For this review, take the finished solid that the model builds, in its own axes (mm). Face numbers are marked on the shaded views. A direction names the side the tool comes from. Round coordinates to 2 decimals unless told otherwise and drop trailing zeros. Loops run counter-clockwise (first coordinate to the right, second up) from the corner with the lowest first, then second, coordinate; pieces in that order, holes last.
1. Tool access review of the marked faces 1, 2 and 3: name each direction out of +Z, -Z, +X, -X, +Y, -Y from which nothing blocks a thin tool from reaching the whole face with its end or side.
2. Clearance check with flat-ended pins moving along their axes: pin 1 Ø1 at (x, y) = (-14.5, 4.5) entering from +Z; pin 2 Ø0.6 at (x, z) = (8, -15.5) entering from +Y; pin 3 Ø12 at (x, z) = (2.5, 13) entering from +Y. State where each tip first meets the part, or that it passes through.
3. Consider section A-A on z = 17.5. State the section outline as (x, y) points, then the cut area to 3 significant figures.
4. To check wall thickness, follow line 1 along X through (y, z) = (18, -0.5); line 2 along Y through (x, z) = (9, 11); line 3 along X through (y, z) = (3.35, 17.5). State the ranges of each line that lie inside material, in increasing order.
5. Consider section D-D on z = -17.5. State how many separate pieces and enclosed holes the cut face has, then the cut area to 3 significant figures.
6. Consider section C-C on z = 5.5. State the section outline as (x, y) points.
7. Draft analysis for pull direction X (two halves, no side actions). For the marked faces 4, 5, 6 and 7, state which applies: released by +X, released by -X, zero draft, split by the parting line, or undercut.
8. Consider section B-B on y = 2.5. State the section outline as (x, z) points, then the cut area to 3 significant figures.
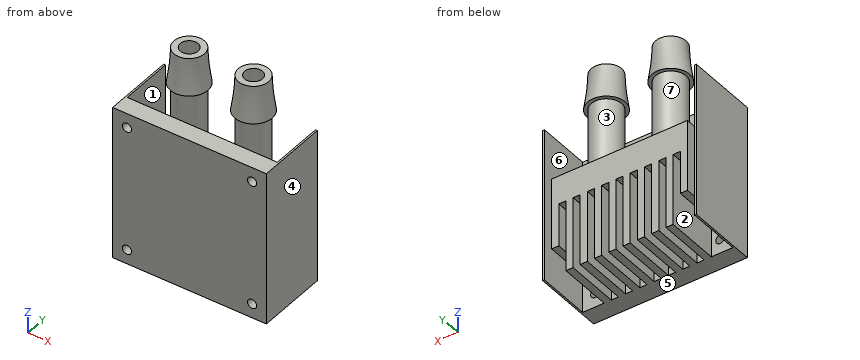
from build123d import *

# Parameters (mm, degrees)
SKETCH1_W               = 43
SKETCH1_H               = 43
BOSS_EXTRUDE1_DEPTH     = 20
SKETCH2_W               = 2
SKETCH2_H               = 15
CUT_EXTRUDE1_DEPTH      = 20
LPATTERN1_COUNT         = 6
LPATTERN1_PITCH         = 4
MIRROR1_COPY_1_SKETCH_W = 2
MIRROR1_COPY_1_SKETCH_H = 15
MIRROR1_COPY_1_DEPTH    = 20
MIRROR1_COPY_2_SKETCH_W = 2
MIRROR1_COPY_2_SKETCH_H = 15
MIRROR1_COPY_2_DEPTH    = 20
MIRROR1_COPY_3_SKETCH_W = 2
MIRROR1_COPY_3_SKETCH_H = 15
MIRROR1_COPY_3_DEPTH    = 20
MIRROR1_COPY_4_SKETCH_W = 2
MIRROR1_COPY_4_SKETCH_H = 15
MIRROR1_COPY_4_DEPTH    = 20
MIRROR1_COPY_5_SKETCH_W = 2
MIRROR1_COPY_5_SKETCH_H = 15
MIRROR1_COPY_5_DEPTH    = 20
MIRROR1_COPY_6_SKETCH_W = 2
MIRROR1_COPY_6_SKETCH_H = 15
MIRROR1_COPY_6_DEPTH    = 20
SKETCH7_W               = 2
SKETCH7_H               = 15
CUT_EXTRUDE6_DEPTH      = 38.299463803
SKETCH8_W               = 38
SKETCH8_H               = 15
CUT_EXTRUDE7_DEPTH      = 15
SKETCH9_R               = 4.25
BOSS_EXTRUDE2_DEPTH     = 20
SKETCH12_R              = 2.5
CUT_EXTRUDE8_DEPTH      = 35
SKETCH13_R              = 1.27
CUT_EXTRUDE9_DEPTH      = 47.845490789
SKETCH14_W              = 2
SKETCH14_H              = 8
CUT_EXTRUDE10_DEPTH     = 15


with BuildPart() as part:
    # Sketch1 → Boss-Extrude1 (new body)
    with BuildSketch(Plane(origin=(0, 0, 0), x_dir=(1, 0, 0), z_dir=(0, 1, 0))):
        Rectangle(SKETCH1_W, SKETCH1_H)
    extrude(amount=BOSS_EXTRUDE1_DEPTH)

    # Sketch2 → Cut-Extrude1 (cut)
    with BuildSketch(Plane(origin=(0, 0, -21.5), x_dir=(-1, 0, 0), z_dir=(0, 0, -1))):
        with Locations((0, 12.5)):
            Rectangle(SKETCH2_W, SKETCH2_H)
    cut_extrude1 = extrude(amount=-CUT_EXTRUDE1_DEPTH, mode=Mode.SUBTRACT)

    # LPattern1: Cut-Extrude1 ×6
    with Locations(*[(i * LPATTERN1_PITCH, 0, 0) for i in range(1, LPATTERN1_COUNT)]):
        add(cut_extrude1, mode=Mode.SUBTRACT)

    # Mirror1 copy 1 sketch → Mirror1 copy 1 (cut)
    with BuildSketch(Plane(origin=(-4, 0, -21.5), x_dir=(1, 0, 0), z_dir=(0, 0, -1))):
        with Locations((0, -12.5)):
            Rectangle(MIRROR1_COPY_1_SKETCH_W, MIRROR1_COPY_1_SKETCH_H)
    extrude(amount=-MIRROR1_COPY_1_DEPTH, mode=Mode.SUBTRACT)

    # Mirror1 copy 2 sketch → Mirror1 copy 2 (cut)
    with BuildSketch(Plane(origin=(-8, 0, -21.5), x_dir=(1, 0, 0), z_dir=(0, 0, -1))):
        with Locations((0, -12.5)):
            Rectangle(MIRROR1_COPY_2_SKETCH_W, MIRROR1_COPY_2_SKETCH_H)
    extrude(amount=-MIRROR1_COPY_2_DEPTH, mode=Mode.SUBTRACT)

    # Mirror1 copy 3 sketch → Mirror1 copy 3 (cut)
    with BuildSketch(Plane(origin=(-12, 0, -21.5), x_dir=(1, 0, 0), z_dir=(0, 0, -1))):
        with Locations((0, -12.5)):
            Rectangle(MIRROR1_COPY_3_SKETCH_W, MIRROR1_COPY_3_SKETCH_H)
    extrude(amount=-MIRROR1_COPY_3_DEPTH, mode=Mode.SUBTRACT)

    # Mirror1 copy 4 sketch → Mirror1 copy 4 (cut)
    with BuildSketch(Plane(origin=(-16, 0, -21.5), x_dir=(1, 0, 0), z_dir=(0, 0, -1))):
        with Locations((0, -12.5)):
            Rectangle(MIRROR1_COPY_4_SKETCH_W, MIRROR1_COPY_4_SKETCH_H)
    extrude(amount=-MIRROR1_COPY_4_DEPTH, mode=Mode.SUBTRACT)

    # Mirror1 copy 5 sketch → Mirror1 copy 5 (cut)
    with BuildSketch(Plane(origin=(-20, 0, -21.5), x_dir=(1, 0, 0), z_dir=(0, 0, -1))):
        with Locations((0, -12.5)):
            Rectangle(MIRROR1_COPY_5_SKETCH_W, MIRROR1_COPY_5_SKETCH_H)
    extrude(amount=-MIRROR1_COPY_5_DEPTH, mode=Mode.SUBTRACT)

    # Mirror1 copy 6 sketch → Mirror1 copy 6 (cut)
    with BuildSketch(Plane(origin=(0, 0, -21.5), x_dir=(1, 0, 0), z_dir=(0, 0, -1))):
        with Locations((0, -12.5)):
            Rectangle(MIRROR1_COPY_6_SKETCH_W, MIRROR1_COPY_6_SKETCH_H)
    extrude(amount=-MIRROR1_COPY_6_DEPTH, mode=Mode.SUBTRACT)

    # Sketch7 → Cut-Extrude6 (cut, through all)
    with BuildSketch(Plane(origin=(0, 0, -1.5), x_dir=(-1, 0, 0), z_dir=(0, 0, -1))):
        with Locations((20, 12.5)):
            Rectangle(SKETCH7_W, SKETCH7_H)
        with Locations((-20, 12.5)):
            Rectangle(SKETCH7_W, SKETCH7_H)
    extrude(amount=-CUT_EXTRUDE6_DEPTH, mode=Mode.SUBTRACT)

    # Sketch8 → Cut-Extrude7 (cut)
    with BuildSketch(Plane.XY.offset(21.5)):
        with Locations((0, 12.5)):
            Rectangle(SKETCH8_W, SKETCH8_H)
    extrude(amount=-CUT_EXTRUDE7_DEPTH, mode=Mode.SUBTRACT)

    # Sketch9 → Boss-Extrude2 (add)
    with BuildSketch(Plane.XY.offset(6.5)):
        with Locations((-9, 12.5)):
            Circle(SKETCH9_R)
    boss_extrude2 = extrude(amount=BOSS_EXTRUDE2_DEPTH)

    # Loft1: read off the stored shape, not the designer's step
    # Loft1: loft between two sections, ruled curve by curve
    loft1_from = [
        Edge.make_bspline([(-10.350301356, 17.57338016, 26.5), (-20.497061676, 14.872777448, 26.5), (-17.796458964, 4.726017128, 26.5), (-7.649698644, 7.42661984, 26.5), (2.497061676, 10.127222552, 26.5), (-0.203541036, 20.273982872, 26.5), (-10.350301356, 17.57338016, 26.5)], [0, 0, 0, 0, 0.5, 0.5, 0.5, 1, 1, 1, 1], 3, [1, 0.333333333, 0.333333333, 1, 0.333333333, 0.333333333, 1]),
    ]
    loft1_to = [
        Edge.make_bspline([(-7.69684054, 16.545278164, 36.5), (-15.787396868, 19.151597083, 36.5), (-18.393715787, 11.061040755, 36.5), (-10.30315946, 8.454721836, 36.5), (-2.212603132, 5.848402917, 36.5), (0.393715787, 13.938959245, 36.5), (-7.69684054, 16.545278164, 36.5)], [0, 0, 0, 0, 0.5, 0.5, 0.5, 1, 1, 1, 1], 3, [1, 0.333333333, 0.333333333, 1, 0.333333333, 0.333333333, 1]),
    ]
    loft1 = Solid(Shell([*[Face.make_surface_from_curves(loft1_from[k], loft1_to[k]) for k in range(1)], Face(Wire(loft1_from)), Face(Wire(loft1_to))]))
    add(loft1)

    # Sketch12 → Cut-Extrude8 (cut)
    with BuildSketch(Plane.XY.offset(36.5)):
        with Locations((-9, 12.5)):
            Circle(SKETCH12_R)
    cut_extrude8 = extrude(amount=-CUT_EXTRUDE8_DEPTH, mode=Mode.SUBTRACT)

    # Mirror3: Boss-Extrude2, Loft1, Cut-Extrude8 across plane
    add(boss_extrude2.mirror(Plane(origin=(0, 0, 0), x_dir=(0, 0, 1), z_dir=(1, 0, 0))))
    add(loft1.mirror(Plane(origin=(0, 0, 0), x_dir=(0, 0, 1), z_dir=(1, 0, 0))))
    add(cut_extrude8.mirror(Plane(origin=(0, 0, 0), x_dir=(0, 0, 1), z_dir=(1, 0, 0))), mode=Mode.SUBTRACT)

    # Sketch13 → Cut-Extrude9 (cut, through all)
    with BuildSketch(Plane.XZ):
        with Locations(Location((17.5, 17.5, 0), (0, 0, 270))):
            Circle(SKETCH13_R)
        with Locations(Location((-17.5, 17.5, 0), (0, 0, 270))):
            Circle(SKETCH13_R)
        with Locations(Location((-17.5, -17.5, 0), (0, 0, 270))):
            Circle(SKETCH13_R)
        with Locations(Location((17.5, -17.5, 0), (0, 0, 270))):
            Circle(SKETCH13_R)
    extrude(amount=-CUT_EXTRUDE9_DEPTH, mode=Mode.SUBTRACT)

    # Sketch14 → Cut-Extrude10 (cut)
    with BuildSketch(Plane(origin=(0, 20, 0), x_dir=(1, 0, 0), z_dir=(0, 1, 0))):
        with Locations((-18, 17.5)):
            Rectangle(SKETCH14_W, SKETCH14_H)
        with Locations((18, 17.5)):
            Rectangle(SKETCH14_W, SKETCH14_H)
    extrude(amount=-CUT_EXTRUDE10_DEPTH, mode=Mode.SUBTRACT)


solid = part.part
Resolved:
1. face 1: +Z, -Z, +Y
1. face 2: -Z, +Y
1. face 3: none
2. pin 1: stops at z = 21.5
2. pin 2: stops at y = 5
2. pin 3: stops at y = 16.72
3. outline: (-21.5, 0) - (-18.77, 0) - (-18.77, 5) - (-21, 5) - (-21, 20) - (-21.5, 20) - close; (-16.23, 0) - (16.23, 0) - (16.23, 5) - (-16.23, 5) - close; circle Ø8.5 at (-9, 12.5); circle Ø8.5 at (9, 12.5); (18.77, 0) - (21.5, 0) - (21.5, 20) - (21, 20) - (21, 5) - (18.77, 5) - close; hole circle Ø5 at (-9, 12.5); hole circle Ø5 at (9, 12.5)
3. area: 279 mm2
4. line 1: x = -21.5 to -21, -19 to 19, 21 to 21.5
4. line 2: y = 0 to 5, 8.25 to 10, 15 to 16.75
4. line 3: x = -21.5 to -18.77, -16.23 to 16.23, 18.77 to 21.5
5. separate pieces: 3
5. enclosed holes: 0
5. area: 445 mm2
6. outline: (-21.5, 0) - (21.5, 0) - (21.5, 20) - (21, 20) - (21, 5) - (19, 5) - (19, 20) - (-19, 20) - (-19, 5) - (-21, 5) - (-21, 20) - (-21.5, 20) - close; hole circle Ø5 at (-9, 12.5); hole circle Ø5 at (9, 12.5)
7. face 4: released by +X
7. face 5: zero draft
7. face 6: undercut
7. face 7: undercut
8. outline: (-21.5, -21.5) - (21.5, -21.5) - (21.5, 21.5) - (-21.5, 21.5) - close; hole circle Ø2.54 at (-17.5, -17.5); hole circle Ø2.54 at (-17.5, 17.5); hole circle Ø2.54 at (17.5, -17.5); hole circle Ø2.54 at (17.5, 17.5)
8. area: 1,830 mm2
